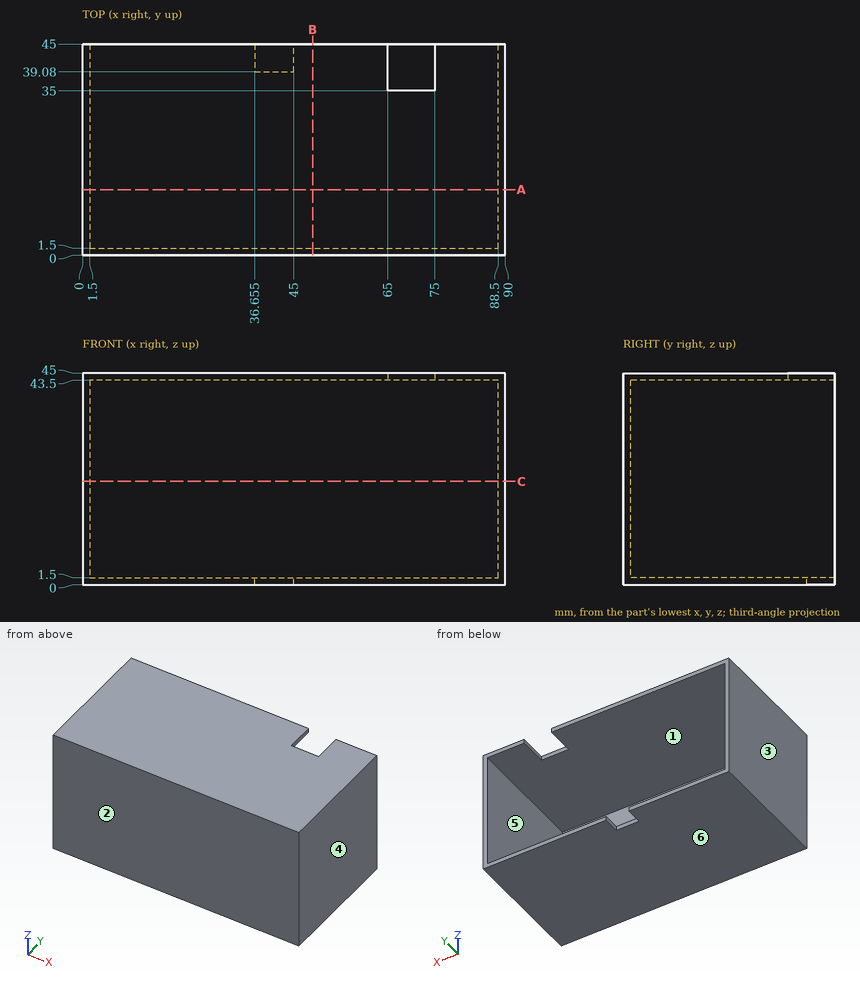
The figure shows three views and two pictorial views of one solid part (mm, origin at its lowest corner). Answer the questions. A direction names the side the tool comes from. Round coordinates to 2 decimals unless told otherwise and drop trailing zeros. Write each loop counter-clockwise with the first axis right and the second up, starting at its lowest first coordinate (ties: lowest second). Pieces come first, ordered by that corner, then holes. Notation, with made-up numbers: M -30,-25.75 L -21,-25.75 A13 cw -21,-20.75 Z; hole C -6.5,64 d10. An arc over 180 degrees is marked long. Use a Markdown table: item, result.
1) The part is cut by section C-C (z = 22). Write down the section's boundary in (x, y).
Answers follow:
| item | result |
|---|---|
| outline | M 0,0 L 90,0 L 90,45 L 88.5,45 L 88.5,1.5 L 1.5,1.5 L 1.5,45 L 0,45 Z |
2) The part is cut by section B-B (x = 49). Write down the section's boundary in (y, z).
Answers follow:
| item | result |
|---|---|
| outline | M 0,0 L 45,0 L 45,1.5 L 1.5,1.5 L 1.5,43.5 L 45,43.5 L 45,45 L 0,45 Z |
3) A tool of negligible diameter and unlimited length cuts with its end or side. For the marked faces 5 and 6, from which of +Z, -Z, +X, -X, +Y, -Y can it reach the whole face along a straight path? Write none if from no direction.
Answers follow:
| item | result |
|---|---|
| face 5 | +Y |
| face 6 | -Z, +X, -X, +Y, -Y |
4) Flat-ended cylindrical pins translate along their axes: pin 1 (5 mm diameter, centred on x = 43, z = 36, fed in from +Y); pin 2 (1.6 mm diameter, centred on x = 42.5, z = 0.5, fed in from +Y). Find the tip coordinate at first contact, or state that the pin passes through.
Answers follow:
| item | result |
|---|---|
| pin 1 | stops at y = 1.5 |
| pin 2 | stops at y = 39.08 |
5) For a pull along X with two mould halves and no side action, classify the marked faces 1, 2, 3 and 4 as pulls with the +X half, pulls with the -X half, needs draft (parallel to the pull), parting line crosses it, or undercut.
Answers follow:
| item | result |
|---|---|
| face 1 | undercut |
| face 2 | needs draft |
| face 3 | pulls with the -X half |
| face 4 | pulls with the +X half |
6) The part is cut by section A-A (y = 14). Write down the section's boundary in (x, z).
Answers follow:
| item | result |
|---|---|
| outline | M 0,0 L 90,0 L 90,45 L 0,45 Z; hole M 1.5,1.5 L 88.5,1.5 L 88.5,43.5 L 1.5,43.5 Z |
7) Straight lines are drawn through the part: line 1 along Z through (x, y) = (25.5, 8.5); line 2 along X through (y, z) = (43, 10); line 3 along Y through (x, z) = (55.5, 38). For each, find the intervals that lie inside material, in ascending order. Write a range as [from, to].
Answers follow:
| item | result |
|---|---|
| line 1 | z = [0, 1.5], [43.5, 45] |
| line 2 | x = [0, 1.5], [88.5, 90] |
| line 3 | y = [0, 1.5] |
